```python
from build123d import *

# Parameters (mm, degrees)
SKETCH_W              = 115
SKETCH_H              = 25
PAD_DEPTH             = 3
PAD001_DEPTH          = 3
SKETCH002_W           = 115
SKETCH002_H           = 25
SKETCH002_W_2         = 96
SKETCH002_H_2         = 3
PAD002_DEPTH          = 3
SKETCH003_R           = 0.825
POCKET_DEPTH          = 245.060315
POLARPATTERN_COUNT    = 2
POLARPATTERN001_COUNT = 2
POLARPATTERN002_COUNT = 2
FILLET_R              = 2
SKETCH004_R           = 12.75
POCKET001_DEPTH       = 3


with BuildPart() as part:
    # Sketch → Pad (new body)
    with BuildSketch(Plane.XY):
        Rectangle(SKETCH_W, SKETCH_H)
    extrude(amount=PAD_DEPTH)

    # Sketch001 (on Face6 of Pad) → Pad001 (join)
    with BuildSketch(Plane.XY.offset(3)):
        Polygon((-57.5, 12.5), (57.5, 12.5), (57.5, 4), (50, 4), (50, 5), (-50, 5), (-50, 4), (-57.5, 4), align=None)
        Polygon((-57.5, -12.5), (57.5, -12.5), (57.5, -4), (50, -4), (50, -5), (-50, -5), (-50, -4), (-57.5, -4), align=None)
    extrude(amount=PAD001_DEPTH)

    # Sketch002 (on Face12 of Pad001) → Pad002 (join)
    with BuildSketch(Plane.XY.offset(6)):
        Rectangle(SKETCH002_W, SKETCH002_H)
        Rectangle(SKETCH002_W_2, SKETCH002_H_2, mode=Mode.SUBTRACT)
    extrude(amount=PAD002_DEPTH)

    # Sketch003 (on Face26 of Pad002) → Pocket (cut, through all)
    with BuildSketch(Plane.XY.offset(9)):
        with Locations((-52.5, 7.5)):
            Circle(SKETCH003_R)
    pocket = extrude(amount=-POCKET_DEPTH, mode=Mode.SUBTRACT)

    # PolarPattern: Pocket ×2 about axis
    polarpattern_axis = Axis((0, 0, 0), (0, 1, 0))
    for i in range(1, POLARPATTERN_COUNT):
        add(pocket.rotate(polarpattern_axis, i * 360 / POLARPATTERN_COUNT), mode=Mode.SUBTRACT)

    # PolarPattern001: Pocket ×2 about axis
    polarpattern001_axis = Axis((0, 0, 0), (1, 0, 0))
    for i in range(1, POLARPATTERN001_COUNT):
        add(pocket.rotate(polarpattern001_axis, i * 360 / POLARPATTERN001_COUNT), mode=Mode.SUBTRACT)

    # PolarPattern002: Pocket ×2 about axis
    polarpattern002_axis = Axis((0, 0, 9), (0, 0, 1))
    for i in range(1, POLARPATTERN002_COUNT):
        add(pocket.rotate(polarpattern002_axis, i * 360 / POLARPATTERN002_COUNT), mode=Mode.SUBTRACT)

    # Fillet
    fillet_edges = [part.edges().sort_by_distance(p)[0] for p in [
        (57.5, 12.5, 7.5),
        (57.5, 12.5, 4.5),
        (57.5, 12.5, 1.5),
        (57.5, -12.5, 7.5),
        (-57.5, 12.5, 7.5),
        (-57.5, -12.5, 7.5),
    ]]
    fillet(fillet_edges, radius=FILLET_R)

    # Sketch004 (on Face2 of Fillet) → Pocket001 (cut)
    with BuildSketch(Plane(origin=(0, 0, 0), x_dir=(1, 0, 0), z_dir=(0, 0, -1))):
        with Locations((0, -4.31247)):
            Circle(SKETCH004_R)
    extrude(amount=-POCKET001_DEPTH, mode=Mode.SUBTRACT)


solid = part.part
```
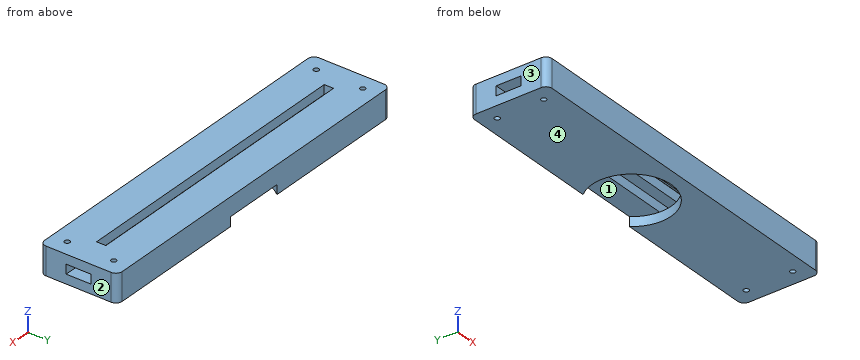
Could you check a few things on this model? Use its own coordinates, in mm. Face numbers are marked on the shaded views. Give positions to 0.01 mm unless a question says otherwise; leave off trailing zeros. Write each loop counter-clockwise with the first axis right and the second up, starting at its lowest first coordinate (ties: lowest second). Pieces come first, ordered by that corner, then holes. Notation, with made-up numbers: (18, 7) - (61, 7) arc R8 cw to (61, 19) - close; hole circle Ø5 at (66, 70). An arc over 180 degrees is marked (long way). One line per item, written item: value. Start each with the question number.
Item 1: Imagine slicing it at B-B, the plane y = 0.5. List the corners of the cut face in (x, z) for me, and give its area (3 significant figures).
Item 2: If we mould it in two halves opening along X, with no side actions, what happens to the marked faces 1, 2, 3 and 4? For each: +X half, -X half, draft (parallel to the pull), parting line (faces both ways), or undercut.
Item 3: Imagine slicing it at D-D, the plane z = 2. List the corners of the cut face in (x, y) for me (3 decimals).
Item 4: Please list where these lines run through material, in increasing order: line 1 (Y direction, x = 52.5, z = 7) (3 decimals); line 2 (Y direction, x = -52.5, z = 5.75) (3 decimals); line 3 (Z direction, x = 15, y = -2). Write a range as from..to.
Item 5: I'm going to push a flat-ended pin straight in: pin 1 (5 mm diameter, centred on x = 6.5, y = 2, fed in from -Z). Where does the tip first touch, or does it pass through?
Item 6: Imagine slicing it at A-A, the plane x = 0. List the corners of the cut face in (y, z) for me.
Item 7: Imagine slicing it at C-C, the plane x = 41.5. List the corners of the cut face in (y, z) for me.
Geometry says:
1. outline: (-57.5, 0) - (-12.17, 0) - (-12.17, 3) - (-57.5, 3) - close; (-57.5, 6) - (-48, 6) - (-48, 9) - (-57.5, 9) - close; (12.17, 0) - (57.5, 0) - (57.5, 3) - (12.17, 3) - close; (48, 6) - (57.5, 6) - (57.5, 9) - (48, 9) - close
1. area: 329 mm^2
2. face 1: undercut
2. face 2: +X half
2. face 3: -X half
2. face 4: draft
3. outline: (-57.5, -10.5) arc R2 ccw to (-55.5, -12.5) - (55.5, -12.5) arc R2 ccw to (57.5, -10.5) - (57.5, 10.5) arc R2 ccw to (55.5, 12.5) - (9.774, 12.5) arc R12.75 cw (long way) to (-9.774, 12.5) - (-55.5, 12.5) arc R2 ccw to (-57.5, 10.5) - close; hole circle Ø1.65 at (-52.5, -7.5); hole circle Ø1.65 at (-52.5, 7.5); hole circle Ø1.65 at (52.5, -7.5); hole circle Ø1.65 at (52.5, 7.5)
4. line 1: -12.5..-8.325, -6.675..6.675, 8.325..12.5
4. line 2: -12.5..-8.325, -6.675..-4, 4..6.675, 8.325..12.5
4. line 3: 0..3, 6..9
5. pin 1: z = 6
6. outline: (-12.5, 0) - (-8.44, 0) - (-8.44, 3) - (-5, 3) - (-5, 6) - (-1.5, 6) - (-1.5, 9) - (-12.5, 9) - close; (1.5, 6) - (5, 6) - (5, 3) - (12.5, 3) - (12.5, 9) - (1.5, 9) - close
7. outline: (-12.5, 0) - (12.5, 0) - (12.5, 9) - (1.5, 9) - (1.5, 6) - (5, 6) - (5, 3) - (-5, 3) - (-5, 6) - (-1.5, 6) - (-1.5, 9) - (-12.5, 9) - close
